Build history of the part. All positions in model axes, mm. Face numbers are marked on the shaded views. A direction names the side the tool comes from. Give positions to 0.01 mm unless a question says otherwise; leave off trailing zeros. Order: outer loops, then holes, each group sorted by start corner. A loop starts at its lowest first (then second) coordinate and runs counter-clockwise, first axis right, second up. Notation, with made-up numbers: (-25.5, 71) - (23.5, 71) arc R14 ccw to (23.5, 86) - close; hole circle Ø9 at (-11, 77.5). An arc over 180 degrees is marked (long way). Answer in a Markdown table with one row per item.
```python
from build123d import *

# Parameters (mm, degrees)
F1_DEPTH = 35.56
F2_R     = 22.86
F3_R     = 3.81
F4_DEPTH = 190.501


with BuildPart() as f1:
    # F0 (on Front) → F1 (new body)
    with BuildSketch(Plane.XZ):
        Polygon((0, 63.5), (0, 0), (12.7, 0), (12.7, 50.8), (177.8, 50.8), (177.8, 0), (190.5, 0), (190.5, 63.5), align=None)
    extrude(amount=F1_DEPTH)

    # F2
    f2_edges = [f1.edges().sort_by_distance(p)[0] for p in [
        (0, -17.78, 63.5),
        (190.5, -17.78, 63.5),
    ]]
    fillet(f2_edges, radius=F2_R)

    # F3 (on face) → F4 (cut, through all)
    with BuildSketch(Plane.YZ.offset(190.5)):
        with Locations((-17.78, 9.841981)):
            Circle(F3_R)
    extrude(amount=-F4_DEPTH, mode=Mode.SUBTRACT)


solid = f1.part
```
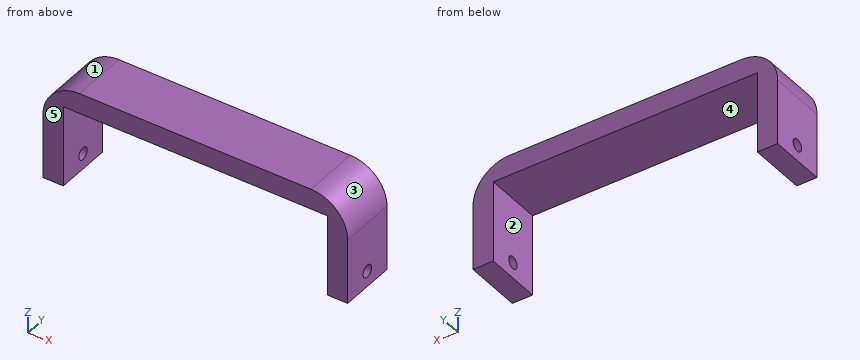
1. Cut at D-D on x = 72. Write the cut outline in (y, z).
Check result:
| item | result |
|---|---|
| outline | (-35.56, 50.8) - (0, 50.8) - (0, 63.5) - (-35.56, 63.5) - close |
2. Cut at C-C on y = -8. Write the cut outline in (x, z), and give its area (3 significant figures).
Check result:
| item | result |
|---|---|
| outline | (0, 0) - (12.7, 0) - (12.7, 50.8) - (177.8, 50.8) - (177.8, 0) - (190.5, 0) - (190.5, 40.64) arc R22.86 ccw to (167.64, 63.5) - (22.86, 63.5) arc R22.86 ccw to (0, 40.64) - close |
| area | 3,490 mm² |
3. Drop flat-ended pins along their axis: P1, Ø12, axis at y = -17.78, z = 9.84, coming from the -X side; P2, Ø6, axis at x = 68.5, y = -20, coming from the -Z side; P3, Ø1, axis at y = -27, z = 57, coming from the -X side. Give the stop position or say it passes through.
Check result:
| item | result |
|---|---|
| P1 | stops at x = 0 |
| P2 | stops at z = 50.8 |
| P3 | stops at x = 6.4 |
4. Two-plate mould, pull along X, no slides. Class the marked faces 3, 4 and 5: +X half, -X half, draft (parallel to the pull), parting line (faces both ways), or undercut.
Check result:
| item | result |
|---|---|
| face 3 | +X half |
| face 4 | undercut |
| face 5 | draft |
5. Probe line 1 (X direction, y = -5, z = 42); line 2 (Z direction, x = 126.5, y = -22); line 3 (X direction, y = -32, z = 46.5). List the from-to ranges inside material, lowest first.
Check result:
| item | result |
|---|---|
| line 1 | x = 0.04 to 12.7, 177.8 to 190.46 |
| line 2 | z = 50.8 to 63.5 |
| line 3 | x = 0.76 to 12.7, 177.8 to 189.74 |
6. Cut at A-A on y = -17.78. Write the cut outline in (x, z).
Check result:
| item | result |
|---|---|
| outline | (0, 0) - (12.7, 0) - (12.7, 6.03) - (0, 6.03) - close; (0, 13.65) - (12.7, 13.65) - (12.7, 50.8) - (177.8, 50.8) - (177.8, 13.65) - (190.5, 13.65) - (190.5, 40.64) arc R22.86 ccw to (167.64, 63.5) - (22.86, 63.5) arc R22.86 ccw to (0, 40.64) - close; (177.8, 0) - (190.5, 0) - (190.5, 6.03) - (177.8, 6.03) - close |
7. Which spindle directions (+Z, -Z, +X, -X, +Y, -Y) get a long thin tool onto all of the face, cutting with end or side? Do the marked faces 1 and 2. Say none if no direction does.
Check result:
| item | result |
|---|---|
| face 1 | +Z, -X, +Y, -Y |
| face 2 | -Z, +Y, -Y |
8. Cut at B-B on z = 28. Write the cut outline in (x, y), and give its area (3 significant figures).
Check result:
| item | result |
|---|---|
| outline | (0, -35.56) - (12.7, -35.56) - (12.7, 0) - (0, 0) - close; (177.8, -35.56) - (190.5, -35.56) - (190.5, 0) - (177.8, 0) - close |
| area | 903 mm² |
